Source: CAD feature listing. Evaluate the final solid. Frame: model axes, mm. A direction names the side the tool comes from. Give positions to 0.01 mm unless a question says otherwise; leave off trailing zeros. Order: outer loops, then holes, each group sorted by start corner. A loop starts at its lowest first (then second) coordinate and runs counter-clockwise, first axis right, second up. Notation, with made-up numbers: M 26,-13.75 L 30,-13.75 A25 cw 30,5.25 Z; hole C 28.5,89.5 d4. An arc over 180 degrees is marked long. Answer in a Markdown table with one row per item. Add a question column.
(1) Material intervals for line 1 along Z through (x, y) = (0, 15); line 2 along X through (y, z) = (22.75, -7); line 3 along Y through (x, z) = (-9.5, -9), sorted ascending.
(2) Section query D-D, the plane z = -10.25. Return loops of the section in (x, y).
(3) Set-up query: faces 5 (the face through (9, 18.986, 0)), 6 (the face through (-9, 18.986, 0)), 7 (the face through (0, 23.749, -3)). Return all of +Z, -Z, +X, -X, +Y, -Y with unobstructed straight access to the full face (end or side cutting, diameter ignored); none if empty.
(4) Section query A-A, the plane z = 0. Return loops of the section in (x, y), plus the area to 3 significant figures.
(5) Section query C-C, the plane y = 17.5. Return loops of the section in (x, z).
(6) Section query B-B, the plane x = 0. Return loops of the section in (y, z).
(7) Mould query, pull axis Z, two halves, no side actions, for faces 1 (the face through (-2.435, 11.708, -0.767)), 2 (the face through (0, 12, 12.7)), 3 (the face through (0, 12, -12.7)), 4 (the face through (-10.922, 9, 0)). Classes: pulls with the +Z half, pulls with the -Z half, needs draft (parallel to the pull), parting line crosses it, or undercut.
(8) Pin query (flat end, axial travel): P1, Ø1.6, axis at x = 10, z = 2, coming from the +Y side; P2, Ø5, axis at y = 22, z = 0, coming from the +X side; P3, Ø4, axis at x = 0, z = 0, coming from the +Y side. Return the tip coordinate at first contact, or that it passes through.
from build123d import *

# Parameters (mm, degrees)
SKETCH1_W                          = 21.844
SKETCH1_H                          = 25.4
BOSS_EXTRUDE1_DEPTH                = 23.749
CLEARANCE_HOLE_FOR_ALIGNMENT_PIN_D = 5.1054
SKETCH6_W                          = 3.140911286
SKETCH6_H                          = 25.4
CLEARANCE_RABBIT_DEPTH             = 4.7625


with BuildPart() as part:
    # Sketch1 → Boss-Extrude1 (new body)
    with BuildSketch(Plane(origin=(0, 0, 0), x_dir=(1, 0, 0), z_dir=(0, 1, 0))):
        Rectangle(SKETCH1_W, SKETCH1_H)
    extrude(amount=BOSS_EXTRUDE1_DEPTH)

    # Clearance Hole for Alignment Pin (through all)
    with Locations(Plane(origin=(0, 23.749, 0), x_dir=(1, 0, 0), z_dir=(0, 1, 0))):
        with Locations((0, 0)):
            Hole(CLEARANCE_HOLE_FOR_ALIGNMENT_PIN_D / 2)

    # Sketch6 → Clearance Rabbit (cut)
    with BuildSketch(Plane(origin=(0, 23.749, 0), x_dir=(1, 0, 0), z_dir=(0, 1, 0))):
        with Locations((9.351544357, 0)):
            Rectangle(SKETCH6_W, SKETCH6_H)
        with Locations((-9.351544357, 0)):
            Rectangle(SKETCH6_W, SKETCH6_H)
    extrude(amount=-CLEARANCE_RABBIT_DEPTH, mode=Mode.SUBTRACT)


solid = part.part
Values follow:
| question | item | result |
|---|---|---|
| 1 | line 1 | z = -12.7 to -2.55, 2.55 to 12.7 |
| 1 | line 2 | x = -7.78 to 7.78 |
| 1 | line 3 | y = 0 to 18.99 |
| 2 | outline | M -10.92,0 L 10.92,0 L 10.92,18.99 L 7.78,18.99 L 7.78,23.75 L -7.78,23.75 L -7.78,18.99 L -10.92,18.99 Z |
| 3 | face 5 | +Z, -Z, +X, +Y |
| 3 | face 6 | +Z, -Z, -X, +Y |
| 3 | face 7 | +Z, -Z, +X, -X, +Y |
| 4 | outline | M -10.92,0 L -2.55,0 L -2.55,23.75 L -7.78,23.75 L -7.78,18.99 L -10.92,18.99 Z; M 2.55,0 L 10.92,0 L 10.92,18.99 L 7.78,18.99 L 7.78,23.75 L 2.55,23.75 Z |
| 4 | area | 368 mm² |
| 5 | outline | M -10.92,-12.7 L 10.92,-12.7 L 10.92,12.7 L -10.92,12.7 Z; hole C 0,0 d5.11 |
| 6 | outline | M 0,-12.7 L 23.75,-12.7 L 23.75,-2.55 L 0,-2.55 Z; M 0,2.55 L 23.75,2.55 L 23.75,12.7 L 0,12.7 Z |
| 7 | face 1 | undercut |
| 7 | face 2 | pulls with the +Z half |
| 7 | face 3 | pulls with the -Z half |
| 7 | face 4 | needs draft |
| 8 | P1 | stops at y = 18.99 |
| 8 | P2 | stops at x = 7.78 |
| 8 | P3 | passes through |
